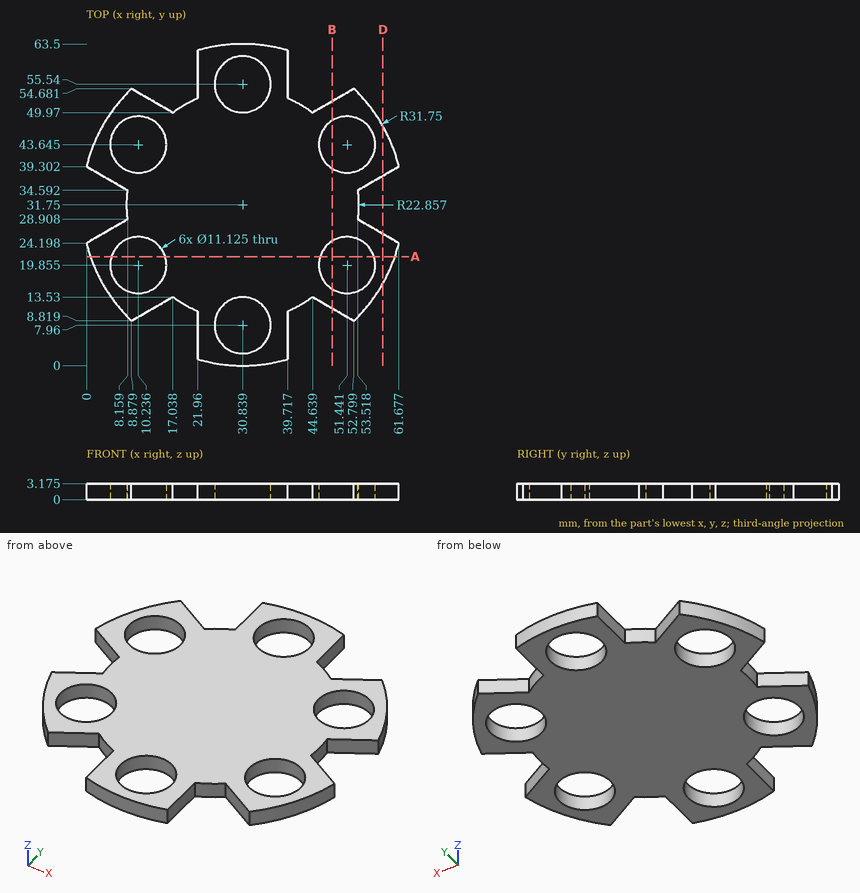
The drawing under review shows one solid part. Ordinate dimensions are in mm from its lowest x, y, z. Round coordinates to 2 decimals unless told otherwise and drop trailing zeros. Loops run counter-clockwise (first coordinate to the right, second up) from the corner with the lowest first, then second, coordinate; pieces in that order, holes last. Notation, with made-up numbers: M -35.5,7.5 L 16.5,7.5 A8 cw 16.5,18.5 Z; hole C 33.25,-16.75 d2. An arc over 180 degrees is marked long. Answer as CSV lines item,"result". Start each with the question number.
Item 1: Consider section A-A (y = 21.5). State how many separate pieces and enclosed holes the cut face has, then the cut area to 3 significant figures.
Item 2: Wall thickness on line 1 (X direction, y = 8, z = 2.5); line 2 (Y direction, x = 27, z = 0.65) (1 decimal); line 3 (X direction, y = 41, z = 2.45) (1 decimal): over which ranges is each line inside the solid? List them lowest first. Write a range as [from, to].
Item 3: Consider section B-B (x = 48.5). Write out the cut boundary in (y, z) (1 decimal).
Item 4: Insertion check: P1, Ø1, axis at x = 27, z = 1, coming from the +Y side; P2, Ø18, axis at x = 10.24, y = 19.86, coming from the -Z side; P3, Ø1, axis at x = 23, z = 1, coming from the +Y side; P4, Ø1, axis at y = 5.5, z = 1.5, coming from the -X side. Each pin has a flat end and moves straight along its axis. Give the tip position at first contact, or say it passes through.
Item 5: Consider section D-D (x = 58.5). Write out the cut boundary in (y, z) (1 decimal).
Answer:
1,separate pieces,"3"
1,enclosed holes,"0"
1,area,"123 mm^2"
2,line 1,"x = [21.96, 25.28], [36.4, 39.72]"
2,line 2,"y = [0.2, 3.9], [12, 51.5], [59.6, 63.3]"
2,line 3,"x = [0.5, 5.3], [15.1, 46.5], [56.3, 61.2]"
3,outline,"M 11.3,0 L 15.1,0 L 15.1,3.2 L 11.3,3.2 Z; M 24.6,0 L 38.9,0 L 38.9,3.2 L 24.6,3.2 Z; M 48.4,0 L 52.2,0 L 52.2,3.2 L 48.4,3.2 Z"
4,P1,"stops at y = 63.32"
4,P2,"stops at z = 0"
4,P3,"stops at y = 62.64"
4,P4,"stops at x = 21.96"
5,outline,"M 16.2,0 L 26,0 L 26,3.2 L 16.2,3.2 Z; M 37.5,0 L 47.3,0 L 47.3,3.2 L 37.5,3.2 Z"
